```python
from build123d import *

# Parameters (mm, degrees)
F0_W     = 63.5
F0_H     = 50.8
F1_DEPTH = 25.4
F2_R     = 12.7
F3_DEPTH = 25.401
F4_R     = 16.51
F4_R_2   = 12.7
F5_DEPTH = 17.018


with BuildPart() as f1:
    # F0 (on Front) → F1 (new body)
    with BuildSketch(Plane.XZ):
        with Locations((-0.3941375762, -5.669991883)):
            Rectangle(F0_W, F0_H)
    extrude(amount=F1_DEPTH)

    # F2 (on face) → F3 (cut, through all)
    with BuildSketch(Plane.XZ.offset(25.4)):
        with Locations((0, -6.3062068075)):
            Circle(F2_R)
    extrude(amount=-F3_DEPTH, mode=Mode.SUBTRACT)

    # F4 (on face) → F5 (join)
    with BuildSketch(Plane.XZ.offset(25.4)):
        with Locations((0, -6.3062068075)):
            Circle(F4_R)
        with Locations((0, -6.3062068075)):
            Circle(F4_R_2, mode=Mode.SUBTRACT)
    extrude(amount=F5_DEPTH)


solid = f1.part
```
Read the model definition and answer for the solid it produces. Units are mm, in the model's axes. A direction names the side the tool comes from. Give positions to 0.01 mm unless a question says otherwise; leave off trailing zeros. Loops run counter-clockwise (first coordinate to the right, second up) from the corner with the lowest first, then second, coordinate; pieces in that order, holes last.
Item 1: Each of these flat-tipped pins is pushed along its axis until it touches: pin 1 Ø3 at (x, y) = (-13.5, -28) entering from +Z; pin 2 Ø6 at (x, z) = (8.5, -17.5) entering from +Y; pin 3 Ø1.5 at (y, z) = (-32.5, 6.5) entering from -X. Where does it stop, or does it pass through?
Item 2: The part is cut by section A-A (x = 0). Write down the section's boundary in (y, z).
Item 3: Find the intervals of material crossed by line 1 along Z through (x, y) = (0, -9.75); line 2 along Z through (x, y) = (0, -37); line 3 along Y through (x, z) = (-27, -2), in increasing order.
Item 4: The part is cut by section D-D (z = 12.5). Write down the section's boundary in (x, y).
Item 5: For faces 1 (the flat face through (-1, -25.4, 12)), 2 (the flat face through (-1, -13, 19.73)), determine the directions among +Z, -Z, +X, -X, +Y, -Y from which every point of the face is accessible in a straight line to the end or side of a thin tool.
Item 6: The part is cut by section C-C (y = -5). Write down the section's boundary in (x, z).
Item 7: The part is cut by section B-B (z = -13.5). Write down the section's boundary in (x, y).
Taken from the geometry:
1. pin 1: stops at z = 5.03
1. pin 2: stops at y = 0
1. pin 3: stops at x = -11.28
2. outline: (-42.42, -22.82) - (-25.4, -22.82) - (-25.4, -31.07) - (0, -31.07) - (0, -19.01) - (-42.42, -19.01) - close; (-42.42, 6.39) - (0, 6.39) - (0, 19.73) - (-25.4, 19.73) - (-25.4, 10.2) - (-42.42, 10.2) - close
3. line 1: z = -31.07 to -19.01, 6.39 to 19.73
3. line 2: z = -22.82 to -19.01, 6.39 to 10.2
3. line 3: y = -25.4 to 0
4. outline: (-32.14, -25.4) - (31.36, -25.4) - (31.36, 0) - (-32.14, 0) - close
5. face 1: -Y
5. face 2: +Z, +X, -X, +Y, -Y
6. outline: (-32.14, -31.07) - (31.36, -31.07) - (31.36, 19.73) - (-32.14, 19.73) - close; hole circle Ø25.4 at (0, -6.31)
7. outline: (-32.14, -25.4) - (-14.86, -25.4) - (-14.86, -42.42) - (-10.47, -42.42) - (-10.47, 0) - (-32.14, 0) - close; (10.47, -42.42) - (14.86, -42.42) - (14.86, -25.4) - (31.36, -25.4) - (31.36, 0) - (10.47, 0) - close
